from build123d import *

# Parameters (mm, degrees)
F1_DEPTH = 30
F0_W     = 15.3
F0_H     = 3.7354312371
F0_W_2   = 15.5
F0_H_2   = 3.2645687629
F0_W_3   = 15.2
F2_DEPTH = 5
F3_W     = 100
F3_H     = 60
F3_W_2   = 92
F3_H_2   = 13
F3_H_3   = 33
F4_DEPTH = 25
F6_DEPTH = 25
F5_W     = 46
F5_H     = 13
F7_DEPTH = 25


with BuildPart() as f1:
    # F0 (on Top) → F1 (new body)
    with BuildSketch(Plane.XY):
        Polygon((0, -30), (50, -30), (50, -10), (18.90296489, -10), (0, -10), (0, -13), (46, -13), (46, -26), (0, -26), align=None)
        Polygon((-50, -30), (0, -30), (0, -26), (-46, -26), (-46, -13), (0, -13), (0, -10), (-50, -10), align=None)
        Polygon((18.90296489, -10), (50, -10), (50, 11.9792576879), (46, 11.9792576879), (46, 6.5132789314), (46, 0), (46, -3.7354312371), (46, -7), (30.5, -7), (18.90296489, -7), align=None)
        Polygon((46, 11.9792576879), (50, 11.9792576879), (50, 30), (-14.5761566237, 30), (-14.5761566237, 26), (0, 26), (15.2, 26), (30.5, 26), (46, 26), (46, 19.4), (46, 12.8), align=None)
        Polygon((0, -10), (18.90296489, -10), (18.90296489, -7), (15.2, -7), (0, -7), (-15.4, -7), (-30.7, -7), (-46, -7), (-46, -3.7354312371), (-46, 0), (-46, 6.5132789314), (-50, 6.5132789314), (-50, -10), align=None)
        Polygon((-50, 30), (-50, 6.5132789314), (-46, 6.5132789314), (-46, 12.8), (-46, 19.4), (-46, 26), (-30.7, 26), (-15.4, 26), (-14.5761566237, 26), (-14.5761566237, 30), align=None)
    extrude(amount=F1_DEPTH)

    # F0 (on Top) → F2 (join)
    with BuildSketch(Plane.XY):
        with BuildLine():
            Line((15.2, 11.5132789314), (15.2, 12.8))
            Line((15.2, 12.8), (0, 12.8))
            Line((0, 12.8), (0, 11.2))
            ThreePointArc((0, 11.2), (3.4229815471, 9.8446120957), (4.99017598, 6.5132789314))
            Line((4.99017598, 6.5132789314), (10.2, 6.5132789314))
            ThreePointArc((10.2, 6.5132789314), (11.6644660941, 10.0488128373), (15.2, 11.5132789314))
        make_face()
        with BuildLine():
            Line((0, 0), (15.2, 0))
            Line((15.2, 0), (15.2, 1.5132789314))
            ThreePointArc((15.2, 1.5132789314), (11.6644660941, 2.9777450254), (10.2, 6.5132789314))
            Line((10.2, 6.5132789314), (4.99017598, 6.5132789314))
            ThreePointArc((4.99017598, 6.5132789314), (4.9975433915, 6.3567164639), (5, 6.2))
            ThreePointArc((5, 6.2), (3.5355339059, 2.6644660941), (0, 1.2))
            Line((0, 1.2), (0, 0))
        make_face()
        with BuildLine():
            Line((0, 12.8), (15.2, 12.8))
            Line((15.2, 12.8), (15.2, 14.4))
            ThreePointArc((15.2, 14.4), (11.6644660941, 15.8644660941), (10.2, 19.4))
            Line((10.2, 19.4), (5, 19.4))
            ThreePointArc((5, 19.4), (3.5355339059, 15.8644660941), (0, 14.4))
            Line((0, 14.4), (0, 12.8))
        make_face()
        with BuildLine():
            Line((15.2, 26), (0, 26))
            Line((0, 26), (0, 24.4))
            ThreePointArc((0, 24.4), (3.5355339059, 22.9355339059), (5, 19.4))
            Line((5, 19.4), (10.2, 19.4))
            ThreePointArc((10.2, 19.4), (11.6644660941, 22.9355339059), (15.2, 24.4))
            Line((15.2, 24.4), (15.2, 26))
        make_face()
        with BuildLine():
            Line((15.2, 0), (30.5, 0))
            Line((30.5, 0), (30.5, 1.2))
            ThreePointArc((30.5, 1.2), (26.8553879043, 2.7770184529), (25.50982402, 6.5132789314))
            Line((25.50982402, 6.5132789314), (20.2, 6.5132789314))
            ThreePointArc((20.2, 6.5132789314), (18.7355339059, 2.9777450254), (15.2, 1.5132789314))
            Line((15.2, 1.5132789314), (15.2, 0))
        make_face()
        with BuildLine():
            Line((30.5, 11.2), (30.5, 12.8))
            Line((30.5, 12.8), (15.2, 12.8))
            Line((15.2, 12.8), (15.2, 11.5132789314))
            ThreePointArc((15.2, 11.5132789314), (18.7355339059, 10.0488128373), (20.2, 6.5132789314))
            Line((20.2, 6.5132789314), (25.50982402, 6.5132789314))
            ThreePointArc((25.50982402, 6.5132789314), (27.0770184529, 9.8446120957), (30.5, 11.2))
        make_face()
        with BuildLine():
            Line((15.2, 12.8), (30.5, 12.8))
            Line((30.5, 12.8), (30.5, 14.4))
            ThreePointArc((30.5, 14.4), (26.9644660941, 15.8644660941), (25.5, 19.4))
            Line((25.5, 19.4), (20.2, 19.4))
            ThreePointArc((20.2, 19.4), (18.7355339059, 15.8644660941), (15.2, 14.4))
            Line((15.2, 14.4), (15.2, 12.8))
        make_face()
        with BuildLine():
            Line((30.5, 26), (15.2, 26))
            Line((15.2, 26), (15.2, 24.4))
            ThreePointArc((15.2, 24.4), (18.7355339059, 22.9355339059), (20.2, 19.4))
            Line((20.2, 19.4), (25.5, 19.4))
            ThreePointArc((25.5, 19.4), (26.9644660941, 22.9355339059), (30.5, 24.4))
            Line((30.5, 24.4), (30.5, 26))
        make_face()
        with BuildLine():
            Line((35.5, 19.4), (46, 19.4))
            Line((46, 19.4), (46, 26))
            Line((46, 26), (30.5, 26))
            Line((30.5, 26), (30.5, 24.4))
            ThreePointArc((30.5, 24.4), (34.0355339059, 22.9355339059), (35.5, 19.4))
        make_face()
        with BuildLine():
            Line((30.5, 12.8), (46, 12.8))
            Line((46, 12.8), (46, 19.4))
            Line((46, 19.4), (35.5, 19.4))
            ThreePointArc((35.5, 19.4), (34.0355339059, 15.8644660941), (30.5, 14.4))
            Line((30.5, 14.4), (30.5, 12.8))
        make_face()
        with BuildLine():
            Line((46, 6.5132789314), (46, 11.9792576879))
            Line((46, 11.9792576879), (46, 12.8))
            Line((46, 12.8), (30.5, 12.8))
            Line((30.5, 12.8), (30.5, 11.2))
            ThreePointArc((30.5, 11.2), (33.9229815471, 9.8446120957), (35.49017598, 6.5132789314))
            Line((35.49017598, 6.5132789314), (46, 6.5132789314))
        make_face()
        with BuildLine():
            Line((46, 0), (46, 6.5132789314))
            Line((46, 6.5132789314), (35.49017598, 6.5132789314))
            ThreePointArc((35.49017598, 6.5132789314), (35.4975433915, 6.3567164639), (35.5, 6.2))
            ThreePointArc((35.5, 6.2), (34.0355339059, 2.6644660941), (30.5, 1.2))
            Line((30.5, 1.2), (30.5, 0))
            Line((30.5, 0), (46, 0))
        make_face()
        with BuildLine():
            Line((-15.4, 0), (0, 0))
            Line((0, 0), (0, 1.2))
            ThreePointArc((0, 1.2), (-3.6446120957, 2.7770184529), (-4.99017598, 6.5132789314))
            Line((-4.99017598, 6.5132789314), (-10.4, 6.5132789314))
            ThreePointArc((-10.4, 6.5132789314), (-11.8644660941, 2.9777450254), (-15.4, 1.5132789314))
            Line((-15.4, 1.5132789314), (-15.4, 0))
        make_face()
        with BuildLine():
            Line((0, 11.2), (0, 12.8))
            Line((0, 12.8), (-15.4, 12.8))
            Line((-15.4, 12.8), (-15.4, 11.5132789314))
            ThreePointArc((-15.4, 11.5132789314), (-11.8644660941, 10.0488128373), (-10.4, 6.5132789314))
            Line((-10.4, 6.5132789314), (-4.99017598, 6.5132789314))
            ThreePointArc((-4.99017598, 6.5132789314), (-3.4229815471, 9.8446120957), (0, 11.2))
        make_face()
        with BuildLine():
            Line((-15.4, 12.8), (0, 12.8))
            Line((0, 12.8), (0, 14.4))
            ThreePointArc((0, 14.4), (-3.5355339059, 15.8644660941), (-5, 19.4))
            Line((-5, 19.4), (-10.4, 19.4))
            ThreePointArc((-10.4, 19.4), (-11.8644660941, 15.8644660941), (-15.4, 14.4))
            Line((-15.4, 14.4), (-15.4, 12.8))
        make_face()
        with BuildLine():
            Line((0, 26), (-14.5761566237, 26))
            Line((-14.5761566237, 26), (-15.4, 26))
            Line((-15.4, 26), (-15.4, 24.4))
            ThreePointArc((-15.4, 24.4), (-11.8644660941, 22.9355339059), (-10.4, 19.4))
            Line((-10.4, 19.4), (-5, 19.4))
            ThreePointArc((-5, 19.4), (-3.5355339059, 22.9355339059), (0, 24.4))
            Line((0, 24.4), (0, 26))
        make_face()
        with BuildLine():
            Line((-15.4, 24.4), (-15.4, 26))
            Line((-15.4, 26), (-30.7, 26))
            Line((-30.7, 26), (-30.7, 24.4))
            ThreePointArc((-30.7, 24.4), (-27.1644660941, 22.9355339059), (-25.7, 19.4))
            Line((-25.7, 19.4), (-20.4, 19.4))
            ThreePointArc((-20.4, 19.4), (-18.9355339059, 22.9355339059), (-15.4, 24.4))
        make_face()
        with BuildLine():
            Line((-46, 26), (-46, 19.4))
            Line((-46, 19.4), (-35.7, 19.4))
            ThreePointArc((-35.7, 19.4), (-34.2355339059, 22.9355339059), (-30.7, 24.4))
            Line((-30.7, 24.4), (-30.7, 26))
            Line((-30.7, 26), (-46, 26))
        make_face()
        with BuildLine():
            Line((-46, 19.4), (-46, 12.8))
            Line((-46, 12.8), (-30.7, 12.8))
            Line((-30.7, 12.8), (-30.7, 14.4))
            ThreePointArc((-30.7, 14.4), (-34.2355339059, 15.8644660941), (-35.7, 19.4))
            Line((-35.7, 19.4), (-46, 19.4))
        make_face()
        with BuildLine():
            Line((-30.7, 14.4), (-30.7, 12.8))
            Line((-30.7, 12.8), (-15.4, 12.8))
            Line((-15.4, 12.8), (-15.4, 14.4))
            ThreePointArc((-15.4, 14.4), (-18.9355339059, 15.8644660941), (-20.4, 19.4))
            Line((-20.4, 19.4), (-25.7, 19.4))
            ThreePointArc((-25.7, 19.4), (-27.1644660941, 15.8644660941), (-30.7, 14.4))
        make_face()
        with BuildLine():
            Line((-15.4, 12.8), (-30.7, 12.8))
            Line((-30.7, 12.8), (-30.7, 11.5132789314))
            ThreePointArc((-30.7, 11.5132789314), (-27.1644660941, 10.0488128373), (-25.7, 6.5132789314))
            Line((-25.7, 6.5132789314), (-20.4, 6.5132789314))
            ThreePointArc((-20.4, 6.5132789314), (-18.9355339059, 10.0488128373), (-15.4, 11.5132789314))
            Line((-15.4, 11.5132789314), (-15.4, 12.8))
        make_face()
        with BuildLine():
            Line((-46, 12.8), (-46, 6.5132789314))
            Line((-46, 6.5132789314), (-35.7, 6.5132789314))
            ThreePointArc((-35.7, 6.5132789314), (-34.2355339059, 10.0488128373), (-30.7, 11.5132789314))
            Line((-30.7, 11.5132789314), (-30.7, 12.8))
            Line((-30.7, 12.8), (-46, 12.8))
        make_face()
        with BuildLine():
            Line((-35.7, 6.5132789314), (-46, 6.5132789314))
            Line((-46, 6.5132789314), (-46, 0))
            Line((-46, 0), (-30.7, 0))
            Line((-30.7, 0), (-30.7, 1.5132789314))
            ThreePointArc((-30.7, 1.5132789314), (-34.2355339059, 2.9777450254), (-35.7, 6.5132789314))
        make_face()
        with BuildLine():
            Line((-30.7, 1.5132789314), (-30.7, 0))
            Line((-30.7, 0), (-15.4, 0))
            Line((-15.4, 0), (-15.4, 1.5132789314))
            ThreePointArc((-15.4, 1.5132789314), (-18.9355339059, 2.9777450254), (-20.4, 6.5132789314))
            Line((-20.4, 6.5132789314), (-25.7, 6.5132789314))
            ThreePointArc((-25.7, 6.5132789314), (-27.1644660941, 2.9777450254), (-30.7, 1.5132789314))
        make_face()
        with Locations((-38.35, -1.8677156186)):
            Rectangle(F0_W, F0_H)
        with Locations((-23.05, -1.8677156186)):
            Rectangle(F0_W, F0_H)
        Polygon((-0.1, -3.7354312371), (0, -3.7354312371), (0, -0.4), (0, 0), (-15.4, 0), (-15.4, -3.7354312371), align=None)
        Polygon((0, -3.7354312371), (15.2, -3.7354312371), (15.2, 0), (0, 0), (0, -0.4), align=None)
        with Locations((22.85, -1.8677156186)):
            Rectangle(F0_W, F0_H)
        with Locations((38.25, -1.8677156186)):
            Rectangle(F0_W_2, F0_H)
        with Locations((-38.35, -5.3677156186)):
            Rectangle(F0_W, F0_H_2)
        with Locations((-23.05, -5.3677156186)):
            Rectangle(F0_W, F0_H_2)
        Polygon((-15.4, -7), (0, -7), (0, -3.7354312371), (-0.1, -3.7354312371), (-15.4, -3.7354312371), align=None)
        with Locations((7.6, -5.3677156186)):
            Rectangle(F0_W_3, F0_H_2)
        Polygon((15.2, -7), (18.90296489, -7), (30.5, -7), (30.5, -3.7354312371), (15.2, -3.7354312371), align=None)
        with Locations((38.25, -5.3677156186)):
            Rectangle(F0_W_2, F0_H_2)
    extrude(amount=F2_DEPTH)

    # F3 (on face) → F4 (join)
    with BuildSketch(Plane.XY.offset(30)):
        Rectangle(F3_W, F3_H)
        with Locations((0, -19.5)):
            Rectangle(F3_W_2, F3_H_2, mode=Mode.SUBTRACT)
        with Locations((0, 9.5)):
            Rectangle(F3_W_2, F3_H_3, mode=Mode.SUBTRACT)
        with Locations((0, 9.5)):
            Rectangle(F3_W_2, F3_H_3)
        with Locations((0, -19.5)):
            Rectangle(F3_W_2, F3_H_2)
    extrude(amount=F4_DEPTH)

    # F5 (on face) → F6 (cut)
    with BuildSketch(Plane.XY.offset(55)):
        with BuildLine():
            ThreePointArc((43.5903112084, 9.5), (29.1903112084, 23.9), (14.7903112084, 9.5))
            Line((14.7903112084, 9.5), (29.1903112084, 9.5))
            Line((29.1903112084, 9.5), (43.5903112084, 9.5))
        make_face()
        with BuildLine():
            Line((29.1903112084, 9.5), (14.7903112084, 9.5))
            ThreePointArc((14.7903112084, 9.5), (29.1903112084, -4.9), (43.5903112084, 9.5))
            Line((43.5903112084, 9.5), (29.1903112084, 9.5))
        make_face()
    extrude(amount=-F6_DEPTH, mode=Mode.SUBTRACT)

    # F5 (on face) → F7 (cut)
    with BuildSketch(Plane.XY.offset(55)):
        with Locations((-23, -19.5)):
            Rectangle(F5_W, F5_H)
        Polygon((-46.0146069527, -10), (-46, -13), (0, -13), (0, -10), align=None)
    extrude(amount=-F7_DEPTH, mode=Mode.SUBTRACT)


solid = f1.part
Design review of the part built by this model. Coordinates are the model's own, in mm. A direction names the side the tool comes from. Coordinates: 2 decimals unless noted, no trailing zeros. Loops run counter-clockwise (first coordinate to the right, second up) from the corner with the lowest first, then second, coordinate; pieces in that order, holes last. Notation, with made-up numbers: M 50.5,-31.5 L 92.5,-31.5 A23 cw 92.5,-19.5 Z; hole C -24,23 d2. An arc over 180 degrees is marked long. Answer as CSV lines item,"result".
Item 1: Add section B-B on z = 44. State the section outline as (x, y) points.
Answer list:
outline,"M -50,-30 L 50,-30 L 50,30 L -50,30 Z; hole M -46.01,-10 L -46,-13 L -46,-26 L 0,-26 L 0,-10 Z; hole C 29.19,9.5 d28.8"
Item 2: Add section A-A on x = -6.5. State the section outline as (y, z) points, plus the area to 4 significant figures.
Answer list:
outline,"M -30,0 L -26,0 L -26,55 L -30,55 Z; M -13,0 L 30,0 L 30,55 L -10,55 L -10,30 L -13,30 Z; hole M -7,5 L 26,5 L 26,30 L -7,30 Z"
area,"1,685 mm²"
Item 3: The part is to be moulded in two halves that separate along Z. For faces 1 (the face through (-46, -20, 28)), 2 (the face through (46, 10, 17)), 3 (the face through (23, -19, 30)), say which applies: pulls with the +Z half, pulls with the -Z half, needs draft (parallel to the pull), parting line crosses it, or undercut.
Answer list:
face 1,"needs draft"
face 2,"undercut"
face 3,"pulls with the -Z half"
Item 4: Add section C-C on y = 3. Count the separate pieces of the cut face and the enclosed holes in it, plus the area to 3 significant figures.
Answer list:
separate pieces,"6"
enclosed holes,"0"
area,"2,370 mm²"
Item 5: For probe 1 along Y at (x, z) = (26.5, 9); probe 2 along Y at (x, z) = (-37, 41.5); probe 3 along X at (y, z) = (9.5, 48.25), list the stretches that pass through material, from the lowest coordinate up.
Answer list:
probe 1,"-30 to -26, -13 to -7, 26 to 30"
probe 2,"-30 to -26, -10 to 30"
probe 3,"-50 to 14.79, 43.59 to 50"
Item 6: Add section D-D on z = 15. State the section outline as (x, y) points, plus the area to 3 significant figures.
Answer list:
outline,"M -50,-30 L 50,-30 L 50,30 L -50,30 Z; hole M -46,-26 L 46,-26 L 46,-13 L -46,-13 Z; hole M -46,-7 L 46,-7 L 46,26 L -46,26 Z"
area,"1,770 mm²"
Item 7: Machinability: for faces 4 (the face through (-1, 0, 55)), 5 (the face through (21.449, -2.642, 42.675)), 6 (the face through (-11, -26, 22)), 7 (the face through (-46, 9, 17)), 8 (the face through (-1, -30, 27)), which of the approach directions +Z, -Z, +X, -X, +Y, -Y give a long, thin tool a straight path to every point of the face, cutting with its end or side? Answer none if there is none.
Answer list:
face 4,"+Z, +X, -X, +Y, -Y"
face 5,"+Z"
face 6,"-Z"
face 7,"none"
face 8,"+Z, -Z, +X, -X, -Y"
Item 8: For P1, Ø1.5, axis at x = 14.5, y = -16.5, coming from the -Z side, flat-tipped, find the tip position at first contact; note if it passes through.
Answer list:
P1,"z = 30"
